Read the model definition and answer for the solid it produces. Units are mm, in the model's axes. Face numbers are marked on the shaded views. Round coordinates to 2 decimals unless told otherwise and drop trailing zeros. Order: outer loops, then holes, each group sorted by start corner. A loop starts at its lowest first (then second) coordinate and runs counter-clockwise, first axis right, second up.
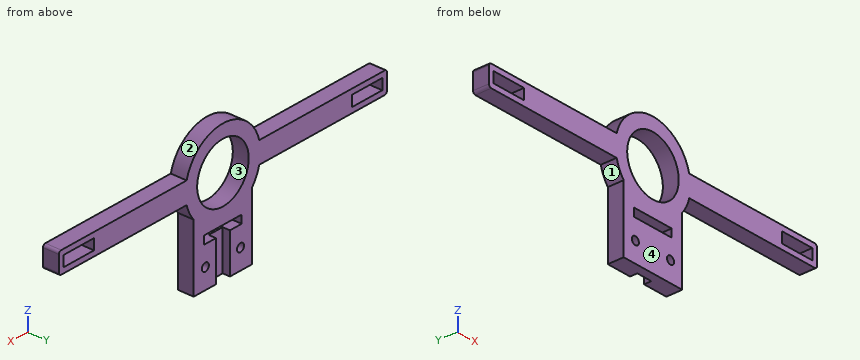
from build123d import *

# Parameters (mm, degrees)
BOX004_W                     = 6
BOX004_H                     = 2.75
BOX004_DEPTH                 = 15
SKETCH023_R                  = 11
SKETCH023_R_2                = 1.5
SKETCH023_W                  = 13
SKETCH023_H                  = 4
SKETCH023_W_2                = 16
SKETCH023_H_2                = 3.01
EXTRUDE015_DEPTH             = 6
CUT002002009_PLACEMENT_ANGLE = 180


with BuildPart() as pendulumclampslot:
    # Box004 → Box004 (new body)
    with BuildSketch(Plane(origin=(-3, 15, -85), x_dir=(1, 0, 0), z_dir=(0, 0, 1))):
        with Locations((3, 1.375)):
            Rectangle(BOX004_W, BOX004_H)
    extrude(amount=BOX004_DEPTH)


with BuildPart() as pendulumclampfront:
    # Sketch023 → Extrude015 (new body)
    with BuildSketch(Plane(origin=(0, 21, -50), x_dir=(1, 0, 0), z_dir=(0, -1, 0))):
        with BuildLine():
            ThreePointArc((-15.491933, -4), (-14.312568, -7.151951), (-12.5, -9.987492))
            Line((-12.5, -35), (-12.5, -9.987492))
            Line((-12.5, -35), (12.5, -35))
            Line((12.5, -35), (12.5, -9.987492))
            ThreePointArc((12.5, -9.987492), (14.312568, -7.151951), (15.491933, -4))
            Line((15.491933, -4), (69, -4))
            ThreePointArc((69, -4), (69.707107, -3.707107), (70, -3))
            Line((70, -3), (70, 3))
            ThreePointArc((70, 3), (69.707107, 3.707107), (69, 4))
            Line((15.491933, 4), (69, 4))
            ThreePointArc((15.491933, 4), (0, 16), (-15.491933, 4))
            Line((-15.491933, 4), (-69, 4))
            ThreePointArc((-69, 4), (-69.707107, 3.707107), (-70, 3))
            Line((-70, 3), (-70, -3))
            ThreePointArc((-70, -3), (-69.707107, -3.707107), (-69, -4))
            Line((-69, -4), (-15.491933, -4))
        make_face()
        Circle(SKETCH023_R, mode=Mode.SUBTRACT)
        with Locations((-7.5, -27.5)):
            Circle(SKETCH023_R_2, mode=Mode.SUBTRACT)
        with Locations((7.5, -27.5)):
            Circle(SKETCH023_R_2, mode=Mode.SUBTRACT)
        with Locations((-61.5, 0)):
            Rectangle(SKETCH023_W, SKETCH023_H, mode=Mode.SUBTRACT)
        with Locations((61.5, 0)):
            Rectangle(SKETCH023_W, SKETCH023_H, mode=Mode.SUBTRACT)
        with Locations((0, -18.495)):
            Rectangle(SKETCH023_W_2, SKETCH023_H_2, mode=Mode.SUBTRACT)
    extrude(amount=EXTRUDE015_DEPTH)

    # Cut002002009: cut PendulumClampSlot
    add(pendulumclampslot.part, mode=Mode.SUBTRACT)


with BuildPart() as pendulumclampfront_1:
    # Cut002002009 placement: moved
    add(pendulumclampfront.part.moved(Location((0, 30, 0))).rotate(Axis((0, 30, 0), (0, 0, 1)), CUT002002009_PLACEMENT_ANGLE))


solid = pendulumclampfront_1.part
Q1. A cutting plane is placed at B-B, the plane x = 0. Give the vertices of the cut face in (y, z).
Outcome:
outline: (9, -85) - (12.25, -85) - (12.25, -70) - (9, -70) - close; (9, -66.99) - (15, -66.99) - (15, -61) - (9, -61) - close; (9, -39) - (15, -39) - (15, -34) - (9, -34) - close
Q2. Flat-ended cylindrical pins translate along their axes: pin 1 (2.5 mm diameter, centred on x = -7.5, z = -77.5, fed in from +Y); pin 2 (1.8 mm diameter, centred on y = 13, z = -75, fed in from -X); pin 3 (3 mm diameter, centred on x = -37, y = 13, fed in from +Z); pin 4 (3 mm diameter, centred on y = 14, z = -75, fed in from +X). Find the tip coordinate at first contact, or state that the pin passes through.
Outcome:
pin 1: passes through
pin 2: stops at x = -12.5
pin 3: stops at z = -46
pin 4: stops at x = 12.5
Q3. For a pull along Z with two mould halves and no side action, classify the marked faces 1, 2, 3 and 4 as released by +Z, released by -Z, zero draft, split by the parting line, or undercut.
Outcome:
face 1: released by -Z
face 2: released by +Z
face 3: undercut
face 4: zero draft
Q4. A cutting plane is placed at C-C, the plane z = -50. Give the vertices of the cut face in (x, y).
Outcome:
outline: (-70, 9) - (-68, 9) - (-68, 15) - (-70, 15) - close; (-55, 9) - (-11, 9) - (-11, 15) - (-55, 15) - close; (11, 9) - (55, 9) - (55, 15) - (11, 15) - close; (68, 9) - (70, 9) - (70, 15) - (68, 15) - close
Q5. A cutting plane is placed at D-D, the plane y = 11.25. Give the number of separate pieces and of enclosed holes in the cut face, plus the area to 3 significant figures.
Outcome:
separate pieces: 1
enclosed holes: 6
area: 1,640 mm2
Q6. Straight lines are drawn through the part: probe 1 along X at (y, z) = (10.75, -77.5); probe 2 along Z at (x, y) = (7.5, 11); probe 3 along X at (y, z) = (12.5, -77.5). For each, find the intervals that lie inside material, in ascending order.
Outcome:
probe 1: x = -12.5 to -9, -6 to 6, 9 to 12.5
probe 2: z = -85 to -79, -76 to -70, -66.99 to -58.05, -41.95 to -35.87
probe 3: x = -12.5 to -9, -6 to -3, 3 to 6, 9 to 12.5
Q7. A cutting plane is placed at A-A, the plane z = -77.5. Give the vertices of the cut face in (x, y).
Outcome:
outline: (-12.5, 9) - (-9, 9) - (-9, 15) - (-12.5, 15) - close; (-6, 9) - (6, 9) - (6, 15) - (3, 15) - (3, 12.25) - (-3, 12.25) - (-3, 15) - (-6, 15) - close; (9, 9) - (12.5, 9) - (12.5, 15) - (9, 15) - close
